```python
from build123d import *

# Parameters (mm, degrees)
F1_DEPTH = 6.35
F3_DEPTH = 6.35
F4_R     = 2.54
F5_R     = 1.27
F6_R     = 0.508


with BuildPart() as f1:
    # F0 (on Top) → F1 (new body)
    with BuildSketch(Plane.XY):
        with BuildLine():
            ThreePointArc((-2.799087249, 39.5839911841), (-0.7915221585, 45.0743154299), (3.4336560515, 41.0342848595))
            Line((3.4336560515, 41.0342848595), (3.3770644537, 36.6740419664))
            Line((3.3770644537, 36.6740419664), (0, -60.1062413045))
            Line((0, -60.1062413045), (11.7469782392, 36.6740419664))
            Line((11.7469782392, 36.6740419664), (11.7469782392, 47.7051909764))
            Line((11.7469782392, 47.7051909764), (0, 47.7051909764))
            ThreePointArc((0, 47.7051909764), (-5.3743672697, 44.4126239501), (-4.8820243994, 38.1291201766))
            Line((-4.8820243994, 38.1291201766), (-2.799087249, 39.5839911841))
        make_face()
    extrude(amount=F1_DEPTH)

    # F2 (on face) → F3 (join, through all)
    with BuildSketch(Plane.XY.offset(6.35)):
        Polygon((5.8018137756, 13.2742899137), (-3.6911324753, 25.4240408597), (-4.6918853336, 24.6421241656), (5.6555386255, 11.3987515904), (17.7563995016, 22.714386033), (17.0525390199, 23.7949541362), align=None)
        Polygon((1.969285928, -3.6702293277), (-4.4911685658, 4.5983219759), (-5.6035720791, 3.9593037682), (1.9003850991, -5.644796836), align=None)
        Polygon((16.2817840507, 5.3620055897), (6.8500791917, -3.6702293277), (6.6085731711, -5.6599343058), (17.1492698758, 4.4343222738), align=None)
        Polygon((1.1045974688, -28.4505659699), (1.1734982977, -26.4759984616), (-2.7963442028, -21.3951103577), (-3.7970970611, -22.1770270519), align=None)
        Polygon((9.207060252, -21.7584877759), (4.0716938985, -26.5606195399), (3.8336266245, -28.5219935843), (10.0760985599, -22.6845964633), align=None)
    extrude(amount=-F3_DEPTH)

    # F4
    f4_edges = [f1.edges().sort_by_distance(p)[0] for p in [
        (2.630216, 15.270776, 3.175),
        (9.066239, 14.588131, 3.175),
        (6.608573, -5.659934, 3.175),
        (1.900385, -5.644797, 3.175),
        (1.104597, -28.450566, 3.175),
        (3.833627, -28.521994, 3.175),
    ]]
    fillet(f4_edges, radius=F4_R)

    # F5
    f5_edges = [f1.edges().sort_by_distance(p)[0] for p in [
        (2.699117, 17.245343, 3.175),
        (9.304306, 16.549505, 3.175),
        (6.850079, -3.670229, 3.175),
        (1.969286, -3.670229, 3.175),
        (1.173498, -26.475998, 3.175),
        (4.071694, -26.56062, 3.175),
    ]]
    fillet(f5_edges, radius=F5_R)

    # F6
    f6_edges = [f1.edges().sort_by_distance(p)[0] for p in [
        (0, -60.106241, 3.175),
    ]]
    fillet(f6_edges, radius=F6_R)


solid = f1.part
```
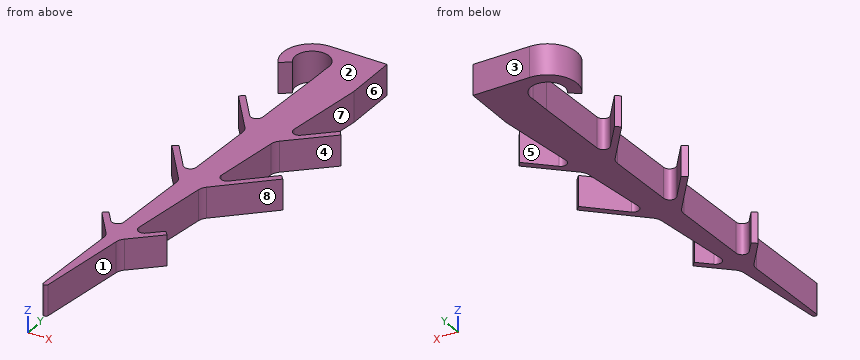
Here's how the part is built. I have some questions about the finished solid (model axes, mm). Face numbers are marked on the shaded views. A direction names the side the tool comes from. Coordinates: 2 decimals unless noted, no trailing zeros. Write each loop counter-clockwise with the first axis right and the second up, starting at its lowest first coordinate (ties: lowest second). Pieces come first, ordered by that corner, then holes. Notation, with made-up numbers: M 37,-23 L 76,-23 A17 ccw 76,-1 Z; hole C 48.25,78 d4. An arc over 180 degrees is marked long. Answer as CSV lines item,"result". Start each with the question number.
Q1. Suppose I cut it at B-B, the plane y = -9. List the corners of the cut face in (x, z) for me, then the cut area to 3 significant figures.
Q2. Will these pins go through, and if not, where does the flat tip stop? pin 1 Ø12 at (x, y) = (5.5, -35.5) entering from -Z; pin 2 Ø4 at (x, y) = (0, 41.67) entering from -Z; pin 3 Ø2 at (y, z) = (-20.5, 2.5) entering from -X; pin 4 Ø2 at (y, z) = (-21.5, 3) entering from +X.
Q3. Suppose I cut it at A-A, the plane x = 15.25. List the corners of the cut face in (y, z) for me, then the cut area to 3 significant figures.
Q4. I need wall thicknesses on probe 1 along Y at (x, z) = (0, 1.5); probe 2 along X at (y, z) = (22, 2.75); probe 3 along X at (y, z) = (3, 0.75). Which ranges of each line are inside material? Lowest first, please. Write a range as [from, to].
Q5. If we mould it in two halves opening along Y, with no side actions, what happens to the marked faces 1, 2, 3 and 4? For each: pulls with the +Y half, pulls with the -Y half, needs draft (parallel to the pull), parting line crosses it, or undercut.
Q6. For the marked faces 5, 6, 7 and 8, which set-ups out of +Z, -Z, +X, -X, +Y, -Y let a thin tool reach every point of the face, with its end or its side?
Entries:
1,outline,"M 1.78,0 L 6.2,0 L 6.2,6.35 L 1.78,6.35 Z"
1,area,"28.1 mm²"
2,pin 1,"stops at z = 0"
2,pin 2,"passes through"
2,pin 3,"stops at x = -2.93"
2,pin 4,"stops at x = 9.9"
3,outline,"M 2.62,0 L 4.37,0 L 4.37,6.35 L 2.62,6.35 Z; M 20.37,0 L 22.11,0 L 22.11,6.35 L 20.37,6.35 Z"
3,area,"22.2 mm²"
4,probe 1,"y = [-27.04, -24.21], [-3.21, -1.11], [18.64, 20.7], [45.17, 47.71]"
4,probe 2,"x = [-2.63, -1.02], [2.87, 9.97], [15.13, 16.99]"
4,probe 3,"x = [-4.85, -3.24], [2.2, 7.66], [13.82, 15.65]"
5,face 1,"pulls with the -Y half"
5,face 2,"needs draft"
5,face 3,"pulls with the +Y half"
5,face 4,"undercut"
6,face 5,"+Z, -Z, +Y"
6,face 6,"+Z, -Z, +X, +Y"
6,face 7,"+Z, -Z"
6,face 8,"+Z, -Z, +X"
